Drawing for the job (mm, zero at the part's lowest x, y, z). A direction names the side the tool comes from. Give positions to 0.01 mm unless a question says otherwise; leave off trailing zeros. Order: outer loops, then holes, each group sorted by start corner. A loop starts at its lowest first (then second) coordinate and runs counter-clockwise, first axis right, second up. Notation, with made-up numbers: (-11.5, -36) - (25.5, -36) arc R10 cw to (25.5, -22) - close; hole circle Ø6 at (43.25, -40). An arc over 180 degrees is marked (long way). Write each question's results on one line, items separated by ' | '. Start each with the question number.
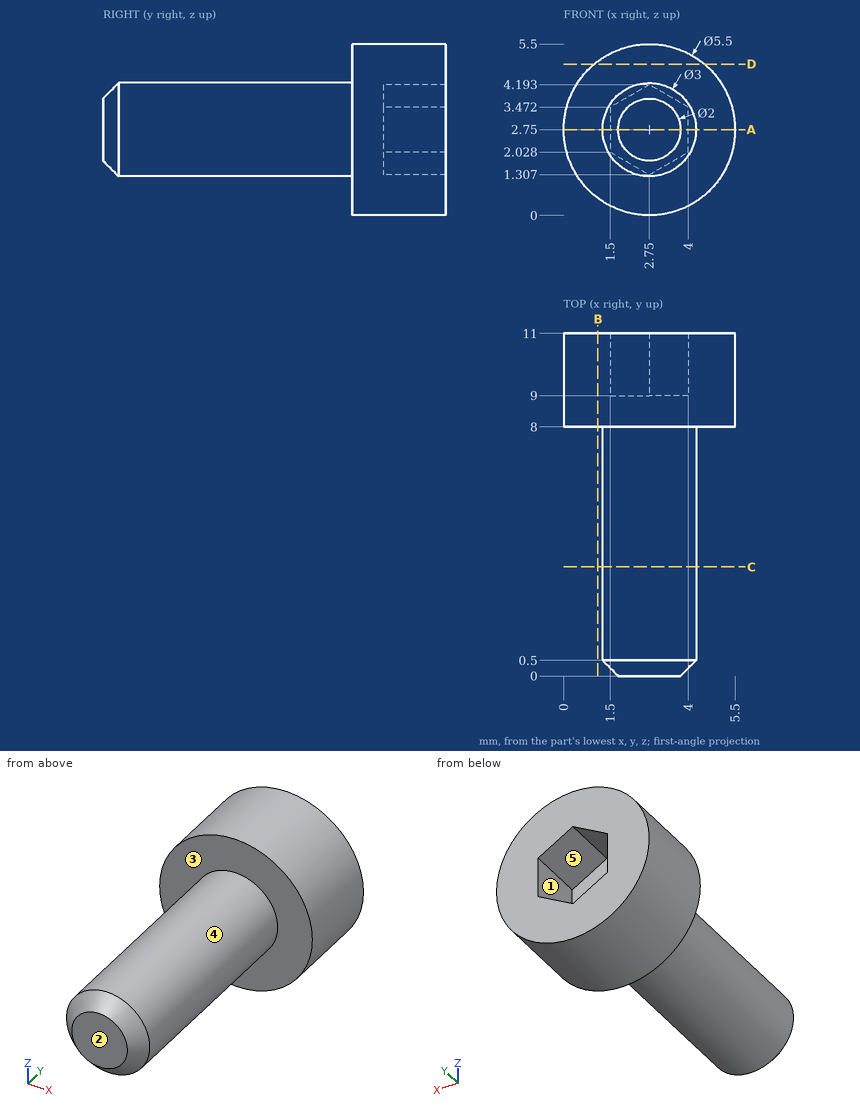
Item 1: Flat gauge pins, fed straight in: pin 1 Ø1 at (x, y) = (1, 3) entering from +Z; pin 2 Ø2 at (x, z) = (1.5, 1) entering from -Y; pin 3 Ø0.7 at (y, z) = (10, 3) entering from -X; pin 4 Ø1.5 at (x, y) = (4.5, 2) entering from +Z. Where does each tip first touch, or does it go through?
Item 2: Cut at C-C, the plane y = 3.5. List the corners of the cut face in (x, z).
Item 3: Cut at B-B, the plane x = 1.1. List the corners of the cut face in (y, z), then the cut area to 3 significant figures.
Item 4: Probe line 1 along Y through (x, z) = (1.55, 4); line 2 along Z through (x, y) = (2.65, 3.5); line 3 along X through (y, z) = (10.5, 1.9) (1 decimal). List the from-to ranges inside material, lowest first. Write a range as from..to.
Item 5: Cut at D-D, the plane z = 4.85. List the corners of the cut face in (x, y) (1 decimal).
Item 6: Two-plate mould, pull along X, no slides. Class the marked faces 3, 4 and 5: +X half, -X half, draft (parallel to the pull), parting line (faces both ways), or undercut.
Item 7: Which spindle directions (+Z, -Z, +X, -X, +Y, -Y) get a long thin tool onto all of the face, cutting with end or side? Do the marked faces 1 and 2. Say none if no direction does.
Item 8: Cut at A-A, the plane z = 2.75. List the corners of the cut face in (x, y).
Values found:
1) pin 1: stops at z = 3.58 | pin 2: stops at y = 0.15 | pin 3: stops at x = 0 | pin 4: stops at z = 3.87
2) outline: circle Ø3 at (2.75, 2.75)
3) outline: (8, 0.55) - (11, 0.55) - (11, 4.95) - (8, 4.95) - close | area: 13.2 mm2
4) line 1: y = 8..11 | line 2: z = 1.25..4.25 | line 3: x = 0.1..1.7, 3.8..5.4
5) outline: (1, 8) - (4.5, 8) - (4.5, 11) - (1, 11) - close
6) face 3: draft | face 4: parting line | face 5: undercut
7) face 1: +Y | face 2: +Z, -Z, +X, -X, -Y
8) outline: (0, 8) - (1.25, 8) - (1.25, 0.5) - (1.75, 0) - (3.75, 0) - (4.25, 0.5) - (4.25, 8) - (5.5, 8) - (5.5, 11) - (4, 11) - (4, 9) - (1.5, 9) - (1.5, 11) - (0, 11) - close
